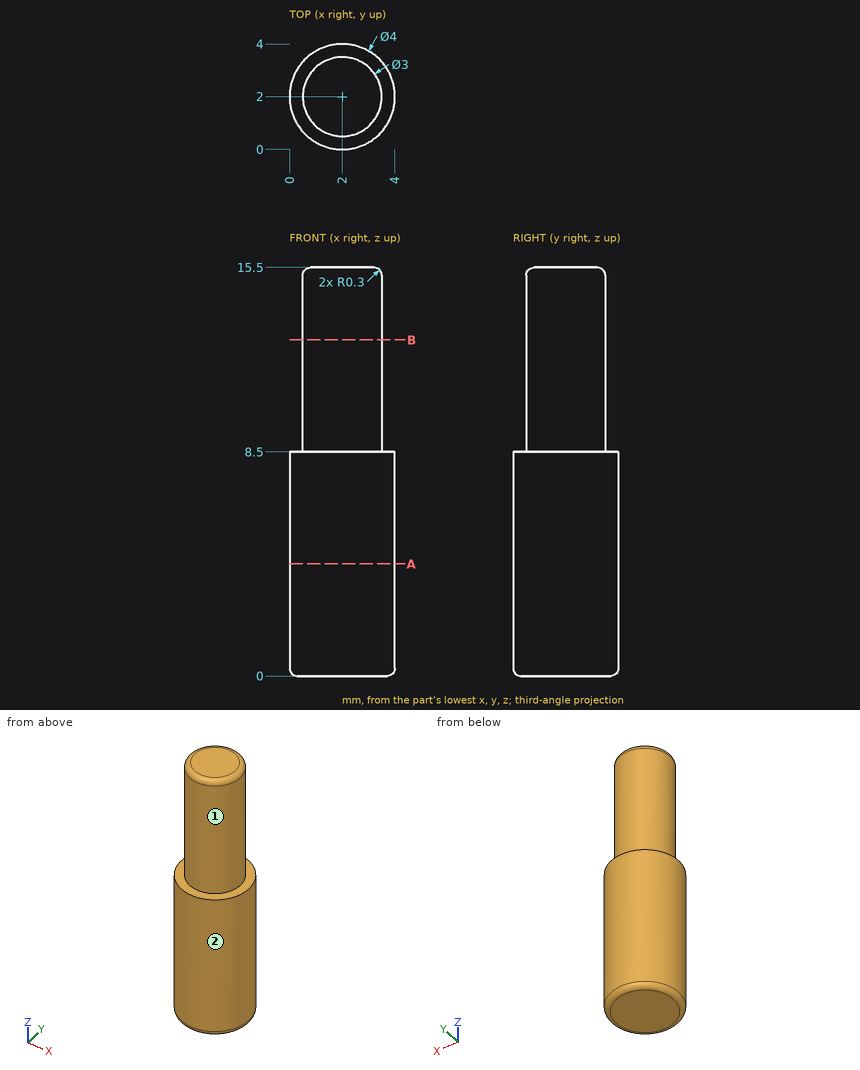
Input: dimensioned drawing with shaded views. Units: mm. Origin: part minimum x, y, z. A direction names the side the tool comes from. Coordinates: 2 decimals unless noted, no trailing zeros. Order: outer loops, then holes, each group sorted by start corner. A loop starts at its lowest first (then second) coordinate and runs counter-clockwise, first axis right, second up.
1. Contact query for a flat-ended pin moving along its axis: P1, Ø1.5, axis at y = 3, z = 11.5, coming from the -X side. Output: stop coordinate, or through.
Checked values:
P1: stops at x = 0.52
2. Cut plane A-A, the plane z = 4.25. Return loops of the section in (x, y), plus the area to 3 significant figures.
Checked values:
outline: circle Ø4 at (2, 2)
area: 12.6 mm2
3. Cut plane B-B, the plane z = 12.75. Return loops of the section in (x, y), plus the area to 3 significant figures.
Checked values:
outline: circle Ø3 at (2, 2)
area: 7.07 mm2
4. Access query for the marked faces 1 and 2. Directions: +Z, -Z, +X, -X, +Y, -Y. A direction counts if a zero-diameter tool reaches every point of the face in a straight line with its end or side. Return the directions, or none.
Checked values:
face 1: +Z
face 2: +Z, -Z
5. Ray query, line 1 along X through (y, z) = (1.1, 9.75); line 2 along Z through (x, y) = (3.15, 1); line 3 along Z through (x, y) = (1.25, 3). Return the intervals inside material, ascending.
Checked values:
line 1: x = 0.8 to 3.2
line 2: z = 0 to 8.5
line 3: z = 0 to 15.5
